Autodesk Inventor part; units mm, degrees
ref_plane "YZ Plane" through (0, 0, 0) normal (1, 0, 0) x (0, 1, 0)
ref_plane "XZ Plane" through (0, 0, 0) normal (0, 1, 0) x (-1, 0, 0)
ref_plane "XY Plane" through (0, 0, 0) normal (0, 0, 1) x (1, 0, 0)
sketch "Sketch1" plane through (0, 0, 0) normal (0, 0, 1) x (1, 0, 0)
  circle A0 centre (8.7376, -2.3876) radius 2.032
  circle A1 centre (-8.7376, -2.3876) radius 2.032
  arc A2 (9.5508, 6.3501) -> (10.564, 6.3532) centre (10.0574, 6.3501) ccw
  line L0 (9.5508, 6.3501) -> (6.3306, 6.3501)
  arc A3 (5.3174, 6.3501) -> (6.3306, 6.3501) centre (5.824, 6.3501) ccw
  line L1 (5.3174, 6.3501) -> (4.2872, 6.3501)
  arc A4 (4.2872, 6.3501) -> (3.2382, 5.3011) centre (4.2872, 5.3011) ccw
  line L2 (3.2382, 5.3011) -> (3.2382, 5.1893)
  arc A5 (3.2382, 5.1893) -> (4.2872, 4.1403) centre (4.2872, 5.1893) ccw
  line L3 (4.2872, 4.1403) -> (6.5409, 4.1403)
  arc A6 (7.2003, 2.5463) -> (6.5409, 4.1403) centre (6.5409, 3.2069) ccw
  line L4 (7.2003, 2.5463) -> (3.8742, -0.7738)
  arc A7 (1.6311, -1.7017) -> (3.8742, -0.7738) centre (1.6311, 1.4733) ccw
  line L5 (1.6311, -1.7017) -> (-1.6318, -1.7017)
  arc A8 (-3.8748, -0.7738) -> (-1.6318, -1.7017) centre (-1.6318, 1.4733) ccw
  line L6 (-3.8748, -0.7738) -> (-7.092, 2.4374)
  arc A9 (-6.3875, 4.1403) -> (-7.092, 2.4374) centre (-6.3875, 3.1432) ccw
  line L7 (-6.3875, 4.1403) -> (-4.2879, 4.1403)
  arc A10 (-4.2879, 4.1403) -> (-3.2388, 5.1893) centre (-4.2879, 5.1893) ccw
  line L8 (-3.2388, 5.1893) -> (-3.2388, 5.3011)
  arc A11 (-3.2388, 5.3011) -> (-4.2879, 6.3501) centre (-4.2879, 5.3011) ccw
  line L9 (-4.2879, 6.3501) -> (-5.3196, 6.3501)
  arc A12 (-6.3328, 6.3501) -> (-5.3196, 6.3501) centre (-5.8262, 6.3501) ccw
  line L10 (-6.3328, 6.3501) -> (-9.5528, 6.3501)
  arc A13 (-10.566, 6.3457) -> (-9.5528, 6.3501) centre (-10.0594, 6.3501) ccw
  line L11 (-10.566, 6.3457) -> (-10.5916, 6.3457)
  arc A14 (-10.5916, 6.3457) -> (-12.7, 4.2373) centre (-10.5916, 4.2373) ccw
  line L12 (-12.7, 4.2373) -> (-12.7, -4.2331)
  arc A15 (-12.7, -4.2331) -> (-10.5647, -6.3413) centre (-10.5916, -4.2331) ccw
  arc A16 (-9.5516, -6.35) -> (-10.5647, -6.3413) centre (-10.0581, -6.3412) ccw
  line L13 (-9.5516, -6.35) -> (-6.323, -6.35)
  arc A17 (-5.31, -6.35) -> (-6.323, -6.35) centre (-5.8165, -6.3412) ccw
  line L14 (-5.31, -6.35) -> (5.31, -6.35)
  arc A18 (6.323, -6.35) -> (5.31, -6.35) centre (5.8165, -6.3412) ccw
  line L15 (6.323, -6.35) -> (9.5502, -6.35)
  arc A19 (10.5633, -6.3403) -> (9.5502, -6.35) centre (10.0567, -6.3412) ccw
  line L16 (10.5633, -6.3403) -> (10.589, -6.3404)
  arc A20 (10.589, -6.3404) -> (12.6991, -4.2321) centre (10.5907, -4.2321) ccw
  line L17 (12.6991, -4.2321) -> (12.6991, 4.2448)
  arc A21 (12.6991, 4.2448) -> (10.5907, 6.3532) centre (10.5907, 4.2448) ccw
  line L18 (10.5907, 6.3532) -> (10.564, 6.3532)
  point P0 (0, 0)
extrude "Extrusion1" add sketch "Sketch1" against normal blind 304.8
properties part number "1050-BLACK-FB"
Check sheet for the modelled part. Datum: model origin and axes. Units: mm. Give positions to 0.01 mm unless a question says otherwise; leave off trailing zeros. Use one line per item in the form item = value. Start each with the question number.
1. Thickness scan on line 1 along X through (y, z) = (-4, -184.5); line 2 along X through (y, z) = (3, -16.5); line 3 along X through (y, z) = (4.25, -116.5). Record the ranges inside material, lowest first. Write a range as from..to.
2. Go/stop test with flat-tipped pins: P1, Ø5, axis at x = 2, z = -149, coming from the +Y side; P2, Ø1, axis at x = 3.5, y = 3, coming from the +Z side; P3, Ø1.6, axis at x = -0.5, z = -213.5, coming from the +Y side; P4, Ø1.5, axis at x = 2, z = -31.5, coming from the +Y side. Record where each tip stops, or that it passes through.
3. Section check A-A (z = -205). Count the separate pieces of the cut face and the enclosed holes in it, and give its area (3 significant figures).
Conclusion:
q1.line_1 = -12.7..-9.97, -7.5..7.5, 9.97..12.7
q1.line_2 = -12.7..-7.37, 7.45..12.7
q1.line_3 = -12.7..-3.82, 3.82..12.7
q2.P1 = 6.35
q2.P2 = through
q2.P3 = -1.7
q2.P4 = -1.5
q3.separate_pieces = 1
q3.enclosed_holes = 2
q3.area = 208 mm²
